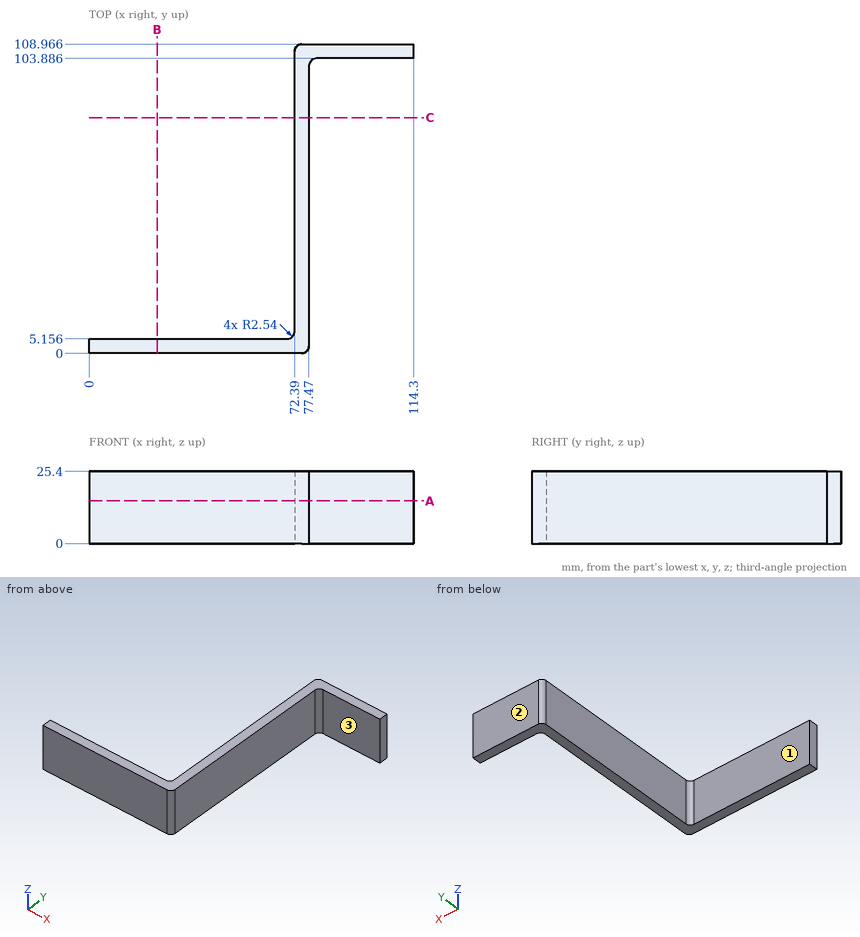
Can you work these out from the drawing? Everything is in mm from the part's minimum corner. A direction names the side the tool comes from. Coordinates: 2 decimals unless noted, no trailing zeros. Order: outer loops, then holes, each group sorted by start corner. A loop starts at its lowest first (then second) coordinate and runs counter-clockwise, first axis right, second up. Notation, with made-up numbers: (11, 40) -> (69, 40) arc R15 cw to (69, 48) -> close; hole circle Ø8 at (-17, 74.5). An arc over 180 degrees is marked (long way). Use one line per item in the form item = value.
Q1. Imagine slicing it at C-C, the plane y = 83. List the corners of the cut face in (x, z) for me, then the cut area to 3 significant figures.
From the geometry:
outline = (72.39, 0) -> (77.47, 0) -> (77.47, 25.4) -> (72.39, 25.4) -> close
area = 129 mm²
Q2. Imagine slicing it at B-B, the plane x = 24. List the corners of the cut face in (y, z) for me, then the cut area to 3 significant figures.
From the geometry:
outline = (0, 0) -> (5.16, 0) -> (5.16, 25.4) -> (0, 25.4) -> close
area = 131 mm²
Q3. I need wall thicknesses on L1, parallel to X at y = 45, z = 10.5; L2, parallel to Y at x = 35.5, z = 3.5; L3, parallel to Y at x = 95, z = 23.75. Which ranges of each line are inside material? Lowest first, please.
From the geometry:
L1 = 72.39 to 77.47
L2 = 0 to 5.16
L3 = 103.89 to 108.97
Q4. Imagine slicing it at A-A, the plane z = 15. List the corners of the cut face in (x, y) for me, then the cut area to 3 significant figures.
From the geometry:
outline = (0, 0) -> (74.93, 0) arc R2.54 ccw to (77.47, 2.54) -> (77.47, 101.35) arc R2.54 cw to (80.01, 103.89) -> (114.3, 103.89) -> (114.3, 108.97) -> (74.93, 108.97) arc R2.54 ccw to (72.39, 106.43) -> (72.39, 7.7) arc R2.54 cw to (69.85, 5.16) -> (0, 5.16) -> close
area = 1,110 mm²
Q5. Will these pins go through, and if not, where does the flat tip stop? P1, Ø6, axis at y = 43, z = 6.5, coming from the -X side; P2, Ø1.5, axis at y = 98, z = 17, coming from the +X side; P3, Ø12.5, axis at x = 42, z = 12, coming from the +Y side.
From the geometry:
P1 = 72.39
P2 = 77.47
P3 = 5.16
Q6. Which directions (+Z, -Z, +X, -X, +Y, -Y) give clear straight access to the entire face, cutting with the end or side of a thin tool? Please do the marked faces 1, 2 and 3.
From the geometry:
face_1 = +Z, -Z, -X, +Y
face_2 = +Z, -Z, +X, -X, +Y
face_3 = +Z, -Z, +X, -Y
